Answer from the drawing. Dimensions are ordinates in mm from the lowest x, y and z of the part. Round coordinates to 2 decimals unless told otherwise and drop trailing zeros. Write each loop counter-clockwise with the first axis right and the second up, starting at its lowest first coordinate (ties: lowest second). Pieces come first, ordered by that corner, then holes. Notation, with made-up numbers: (19.25, -27.75) - (63.25, -27.75) arc R30 ccw to (63.25, 5.25) - close; hole circle Ø1 at (87, 20). An arc over 180 degrees is marked (long way). Answer as a JSON object with one key per item and string values.
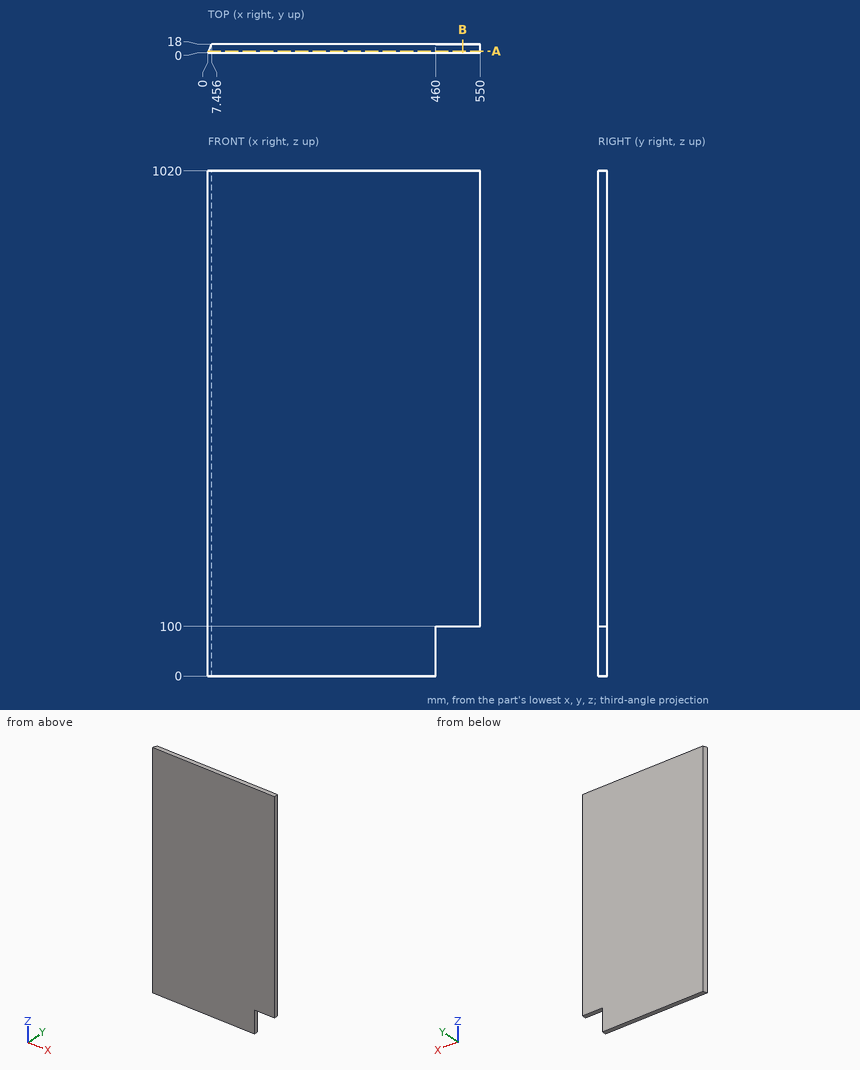
Item 1: Consider line 1 along Z through (x, y) = (504, 2.75); line 2 along X through (y, z) = (13.75, 654.5) (1 decimal); line 3 along X through (y, z) = (17, 779). Determine where each line is inside the solid, lowest interval first.
Results found:
{"line 1": "100 to 1020", "line 2": "5.7 to 550", "line 3": "7.04 to 550"}
Item 2: Each of these flat-tipped pins is pushed along its axis until it touches: P1, Ø10, axis at y = 11, z = 242, coming from the -X side (1 decimal); P2, Ø1, axis at y = 7.5, z = 406.5, coming from the -X side. Where does it stop, or does it pass through?
Results found:
{"P1": "x = 2.5", "P2": "x = 2.9"}
Item 3: A cutting plane is placed at B-B (x = 514.5). Write down the section's boundary in (y, z), and give its area (3 significant figures).
Results found:
{"outline": "(0, 100) - (18, 100) - (18, 1020) - (0, 1020) - close", "area": "16,600 mm²"}
Item 4: A cutting plane is placed at A-A (y = 3.5). Write down the section's boundary in (x, z), and give its area (3 significant figures).
Results found:
{"outline": "(1.45, 0) - (460, 0) - (460, 100) - (550, 100) - (550, 1020) - (1.45, 1020) - close", "area": "551,000 mm²"}
